from build123d import *

# Parameters (mm, degrees)
BOSS_EXTRUDE1_DEPTH = 3.175
SKETCH2_W           = 3.175
SKETCH2_H           = 112.395
BOSS_EXTRUDE2_DEPTH = 3.175
FILLET1_R           = 2.54


with BuildPart() as part:
    # Sketch1 → Boss-Extrude1 (new body)
    with BuildSketch(Plane.XY):
        Polygon((61.2775, 1.5875), (61.2775, -56.1975), (0, -56.1975), (-90.8525, -56.1975), (-90.8525, 5.302053944), (-90.8525, 56.1975), (-7.104289944, 56.1975), (61.2775, 56.1975), align=None)
        Polygon((-73.0725, -29.6525), (-10.985, -29.6525), (51.1025, -29.6525), (51.1025, 9.935), (51.1025, 49.5225), (-10.985, 49.5225), (-73.0725, 49.5225), (-73.0725, 47.935), (-73.0725, 9.935), align=None, mode=Mode.SUBTRACT)
    extrude(amount=BOSS_EXTRUDE1_DEPTH)

    # Sketch2 → Boss-Extrude2 (add)
    with BuildSketch(Plane(origin=(61.2775, 0, 0), x_dir=(0, 0, -1), z_dir=(1, 0, 0))):
        with Locations((-1.5875, 0)):
            Rectangle(SKETCH2_W, SKETCH2_H)
    extrude(amount=BOSS_EXTRUDE2_DEPTH)

    # Fillet1
    fillet1_edges = [part.edges().sort_by_distance(p)[0] for p in [
        (51.1025, -29.6525, 1.5875),
        (51.1025, 49.5225, 1.5875),
        (-73.0725, 49.5225, 1.5875),
        (-73.0725, -29.6525, 1.5875),
    ]]
    fillet(fillet1_edges, radius=FILLET1_R)


solid = part.part
Input: part model. Units: mm. Frame: model coordinates. A direction names the side the tool comes from. Give positions to 0.01 mm unless a question says otherwise; leave off trailing zeros. Loops run counter-clockwise (first coordinate to the right, second up) from the corner with the lowest first, then second, coordinate; pieces in that order, holes last. Notation, with made-up numbers: M 44.25,83 L 50.25,83 A17 ccw 50.25,113 Z; hole C 86.5,65.5 d7. An arc over 180 degrees is marked long. Use CSV: the item, a comma, the result in double quotes.
(1) Material intervals for L1, parallel to X at y = 6, z = 1.45; L2, parallel to Y at x = -34, z = 2.6, sorted ascending. Write a range as [from, to].
Outcome:
L1,"x = [-90.85, -73.07], [51.1, 64.45]"
L2,"y = [-56.2, -29.65], [49.52, 56.2]"
(2) Section C-C, the plane z = 2.1. Return loops of the section in (x, y), plus the area to 3 significant figures.
Outcome:
outline,"M -90.85,-56.2 L 64.45,-56.2 L 64.45,56.2 L -90.85,56.2 Z; hole M -73.07,-27.11 A2.54 ccw -70.53,-29.65 L 48.56,-29.65 A2.54 ccw 51.1,-27.11 L 51.1,46.98 A2.54 ccw 48.56,49.52 L -70.53,49.52 A2.54 ccw -73.07,46.98 Z"
area,"7,630 mm²"
(3) Pull-direction query (X, two-part tool) for faces 1 (the face through (64.452, 1, 2)), 2 (the face through (-14, -38, 0)), 3 (the face through (-73.072, 9, 2)); classes: pulls with the +X half, pulls with the -X half, needs draft (parallel to the pull), parting line crosses it, or undercut.
Outcome:
face 1,"pulls with the +X half"
face 2,"needs draft"
face 3,"undercut"
(4) Pin query (flat end, axial travel): P1, Ø12, axis at x = 45.5, y = 19.5, coming from the +Z side (3 decimals). Return the tip coordinate at first contact, or that it passes through.
Outcome:
P1,"stops at z = 3.175"
(5) Section B-B, the plane x = -59.5. Return loops of the section in (y, z) (1 decimal), plus the area to 3 significant figures.
Outcome:
outline,"M -56.2,0 L -29.7,0 L -29.7,3.2 L -56.2,3.2 Z; M 49.5,0 L 56.2,0 L 56.2,3.2 L 49.5,3.2 Z"
area,"105 mm²"
(6) Set-up query: faces 4 (the face through (-14, 56.198, 2)), 5 (the face through (51.102, 10, 2)). Return all of +Z, -Z, +X, -X, +Y, -Y with unobstructed straight access to the full face (end or side cutting, diameter ignored); none if empty.
Outcome:
face 4,"+Z, -Z, +X, -X, +Y"
face 5,"+Z, -Z"
(7) Section A-A, the plane y = 7.5. Return loops of the section in (x, z) (1 decimal).
Outcome:
outline,"M -90.9,0 L -73.1,0 L -73.1,3.2 L -90.9,3.2 Z; M 51.1,0 L 64.5,0 L 64.5,3.2 L 51.1,3.2 Z"
